from build123d import *

# Parameters (mm, degrees)
SKETCH1_R           = 2.75
BOSS_EXTRUDE1_DEPTH = 10


with BuildPart() as part:
    # Sketch1 → Boss-Extrude1 (new body)
    with BuildSketch(Plane.XY):
        Polygon((7.5, -12.990381057), (2.5, -9.330127019), (0, -15), (-2.5, -9.330127019), (-7.5, -12.990381057), (-6.830127019, -6.830127019), (-12.990381057, -7.5), (-9.330127019, -2.5), (-15, 0), (-9.330127019, 2.5), (-12.990381057, 7.5), (-6.830127019, 6.830127019), (-7.5, 12.990381057), (-2.5, 9.330127019), (0, 15), (2.5, 9.330127019), (7.5, 12.990381057), (6.830127019, 6.830127019), (12.990381057, 7.5), (9.330127019, 2.5), (15, 0), (9.330127019, -2.5), (12.990381057, -7.5), (6.830127019, -6.830127019), align=None)
        Circle(SKETCH1_R, mode=Mode.SUBTRACT)
    extrude(amount=BOSS_EXTRUDE1_DEPTH)


solid = part.part
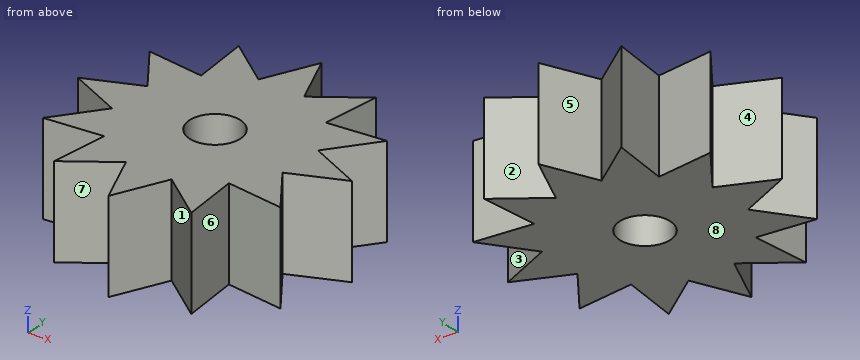
The listing builds one solid part. Answer for the finished solid, in the listing's coordinates (mm). Face numbers are marked on the shaded views. A direction names the side the tool comes from. Round coordinates to 2 decimals unless told otherwise and drop trailing zeros. Write each loop counter-clockwise with the first axis right and the second up, starting at its lowest first coordinate (ties: lowest second). Pieces come first, ordered by that corner, then holes. Notation, with made-up numbers: (-18, -1) - (25, -1) arc R17 ccw to (25, 29) - close; hole circle Ø7 at (-17.5, 32.25). An arc over 180 degrees is marked (long way). Use a Markdown table: item, result. Add a question column.
1. Consider line 1 (Y direction, x = -11.5, z = 4); line 2 (X direction, y = -9.5, z = 4.75); line 3 (Y direction, x = 10, z = 3.5). Determine where each line is inside the solid, lowest interval first.
2. The part is cut by section C-C (y = -10.5). Write down the section's boundary in (x, z).
3. The part is cut by section D-D (x = -6.25). Write down the section's boundary in (y, z).
4. A tool of negligible diameter and unlimited length cuts with its end or side. For the marked faces 1, 2, 3 and 4, from which of +Z, -Z, +X, -X, +Y, -Y can it reach the whole face along a straight path? Write none if from no direction.
5. Flat-ended cylindrical pins translate along their axes: P1, Ø2, axis at y = -7, z = 4, coming from the -X side; P2, Ø5, axis at y = -11, z = 2.5, coming from the -X side; P3, Ø5, axis at x = -2, z = 7, coming from the -Y side; P4, Ø4.5, axis at x = 0, y = 0, coming from the +Z side. Find the tip coordinate at first contact, or state that the pin passes through.
6. The part is cut by section A-A (x = -2). Write down the section's boundary in (y, z).
7. The part is cut by section B-B (z = 1.5). Write down the section's boundary in (x, y), and give its area (3 significant figures).
8. For a pull along Y with two mould halves and no side action, classify the marked faces 5, 6, 7 and 8 as +Y half, -Y half, draft (parallel to the pull), parting line (faces both ways), or undercut.
Reported:
| question | item | result |
|---|---|---|
| 1 | line 1 | -7.34 to -5.46, -1.54 to 1.54, 5.46 to 7.34 |
| 1 | line 2 | -7.12 to -2.73, -2.43 to 2.43, 2.73 to 7.12 |
| 1 | line 3 | -7.17 to -3.42, -2.2 to 2.2, 3.42 to 7.17 |
| 2 | outline | (-7.23, 0) - (-4.1, 0) - (-4.1, 10) - (-7.23, 10) - close; (-1.98, 0) - (1.98, 0) - (1.98, 10) - (-1.98, 10) - close; (4.1, 0) - (7.23, 0) - (7.23, 10) - (4.1, 10) - close |
| 3 | outline | (-12.08, 0) - (12.08, 0) - (12.08, 10) - (-12.08, 10) - close |
| 4 | face 1 | +Z, -Z, -Y |
| 4 | face 2 | +Z, -Z, +Y |
| 4 | face 3 | +Z, -Z, +X |
| 4 | face 4 | +Z, -Z, -X |
| 5 | P1 | x = -12.99 |
| 5 | P2 | x = -7.5 |
| 5 | P3 | y = -15 |
| 5 | P4 | through |
| 6 | outline | (-10.46, 0) - (-1.89, 0) - (-1.89, 10) - (-10.46, 10) - close; (1.89, 0) - (10.46, 0) - (10.46, 10) - (1.89, 10) - close |
| 7 | outline | (-15, 0) - (-9.33, -2.5) - (-12.99, -7.5) - (-6.83, -6.83) - (-7.5, -12.99) - (-2.5, -9.33) - (0, -15) - (2.5, -9.33) - (7.5, -12.99) - (6.83, -6.83) - (12.99, -7.5) - (9.33, -2.5) - (15, 0) - (9.33, 2.5) - (12.99, 7.5) - (6.83, 6.83) - (7.5, 12.99) - (2.5, 9.33) - (0, 15) - (-2.5, 9.33) - (-7.5, 12.99) - (-6.83, 6.83) - (-12.99, 7.5) - (-9.33, 2.5) - close; hole circle Ø5.5 at (0, 0) |
| 7 | area | 426 mm^2 |
| 8 | face 5 | +Y half |
| 8 | face 6 | undercut |
| 8 | face 7 | -Y half |
| 8 | face 8 | draft |
